Input: dimensioned drawing with shaded views. Units: mm. Origin: part minimum x, y, z. A direction names the side the tool comes from. Coordinates: 2 decimals unless noted, no trailing zeros. Order: outer loops, then holes, each group sorted by start corner. A loop starts at its lowest first (then second) coordinate and runs counter-clockwise, first axis right, second up. Notation, with made-up numbers: (44.25, 32) -> (97.25, 32) arc R10 ccw to (97.25, 39) -> close; hole circle Ø1 at (88.5, 23.5). An arc over 180 degrees is marked (long way). Answer as CSV lines item,"result".
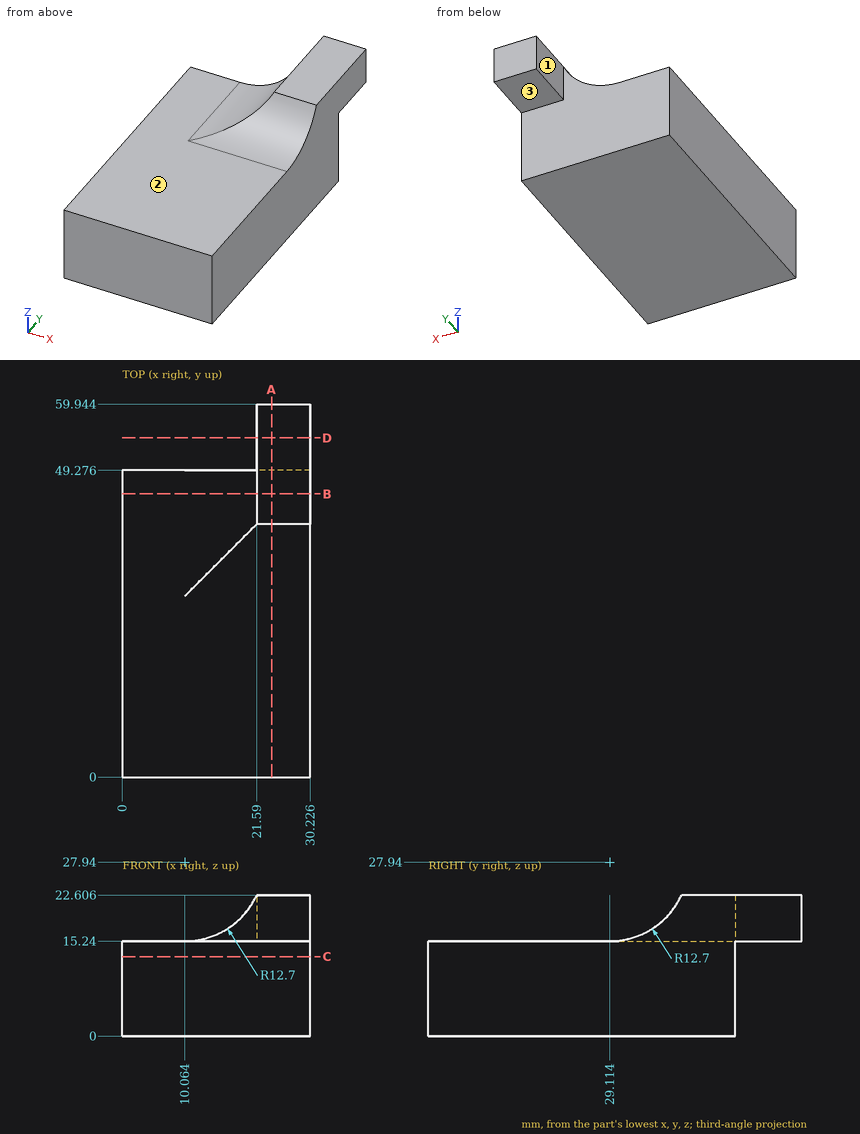
1. Reachability of the marked faces 1, 2 and 3 from +Z, -Z, +X, -X, +Y, -Y: full face, straight path, thin tool, end or side. Return the list, or none.
Findings:
face 1,"+Z, -Z, -X, +Y"
face 2,"+Z, -X, -Y"
face 3,"-Z, +X, -X, +Y"
2. Cut plane D-D (y = 54.5). Return the cut outline in (x, z), plus the area to 3 significant figures.
Findings:
outline,"(21.59, 15.24) -> (30.23, 15.24) -> (30.23, 22.61) -> (21.59, 22.61) -> close"
area,"63.6 mm2"
3. Cut plane A-A (x = 24). Return the cut outline in (y, z) (1 decimal).
Findings:
outline,"(0, 0) -> (49.3, 0) -> (49.3, 15.2) -> (59.9, 15.2) -> (59.9, 22.6) -> (40.6, 22.6) arc R12.7 cw to (29.1, 15.2) -> (0, 15.2) -> close"
4. Ray query, line 1 along X through (y, z) = (53, 21.5); line 2 along Y through (x, z) = (12.5, 6.25); line 3 along Z through (x, y) = (2.5, 19). Return the intervals inside material, ascending.
Findings:
line 1,"x = 21.59 to 30.23"
line 2,"y = 0 to 49.28"
line 3,"z = 0 to 15.24"
5. Cut plane C-C (z = 12.75). Return the cut outline in (x, y).
Findings:
outline,"(0, 0) -> (30.23, 0) -> (30.23, 49.28) -> (0, 49.28) -> close"
6. Contact query for flat-ended pins moving along their axis: pin 1 (1.5 mm diameter, centred on x = 7.5, z = 6.5, fed in from +Y); pin 2 (9 mm diameter, centred on x = 8.5, y = 17, fed in from +Z); pin 3 (6 mm diameter, centred on y = 57, z = 20, fed in from -X). Output: stop coordinate, or through.
Findings:
pin 1,"stops at y = 49.28"
pin 2,"stops at z = 15.24"
pin 3,"stops at x = 21.59"
7. Cut plane B-B (y = 45.5). Return the cut outline in (x, z) (1 decimal), plus the area to 3 significant figures.
Findings:
outline,"(0, 0) -> (30.2, 0) -> (30.2, 22.6) -> (21.6, 22.6) arc R12.7 cw to (10.1, 15.2) -> (0, 15.2) -> close"
area,"548 mm2"
